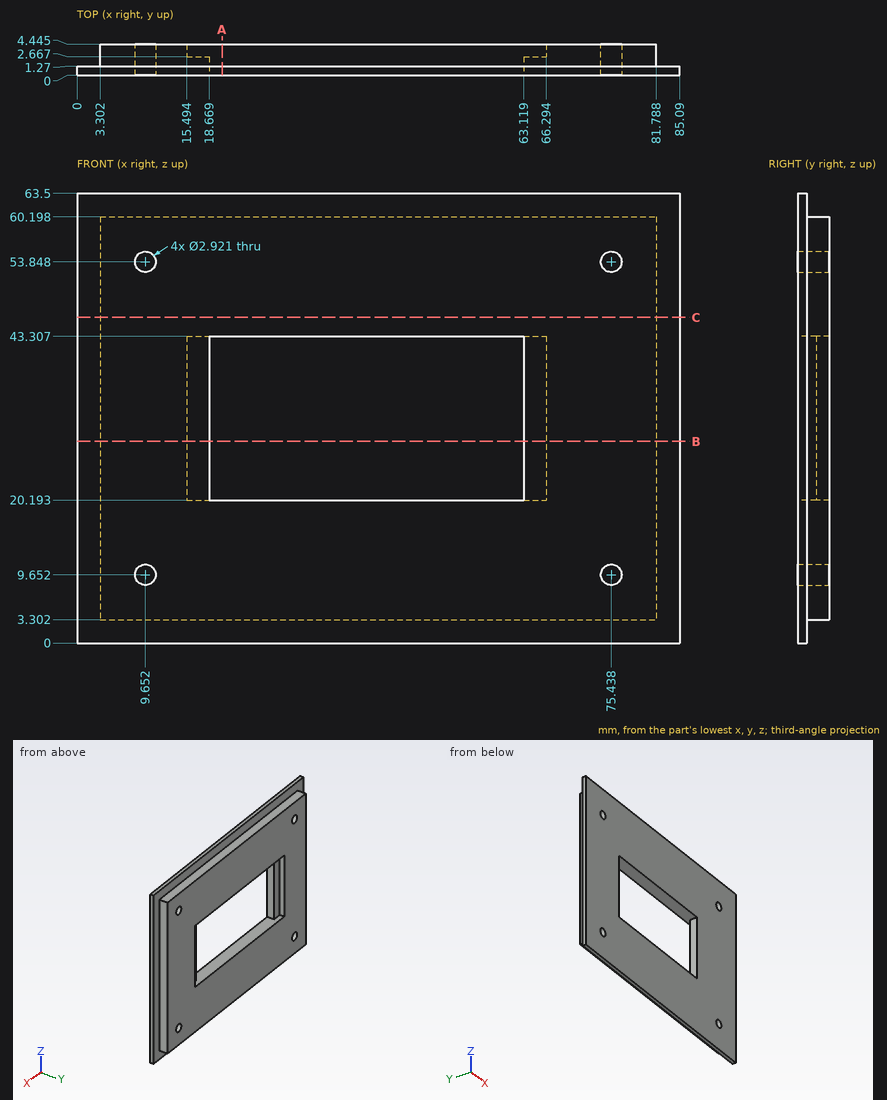
Here's the drawing with two shaded views (mm, measured from the low corner). I have some questions. Coordinates: 2 decimals unless noted, no trailing zeros. Write each loop counter-clockwise with the first axis right and the second up, starting at its lowest first coordinate (ties: lowest second). Pieces come first, ordered by that corner, then holes.
Item 1: I want a section at B-B on z = 28.5. Write out the boundary of the cut face in (x, y) (3 decimals).
Item 2: I want a section at C-C on z = 46. Write out the boundary of the cut face in (x, y) (3 decimals).
Item 3: I want a section at A-A on x = 20.5. Write out the boundary of the cut face in (y, z) (3 decimals).
Item 4: Will these pins go through, and if not, where does the flat tip stop? pin 1 (1.3 mm diameter, centred on x = 46.5, y = 2, fed in from +Z); pin 2 (1.6 mm diameter, centred on x = 65, z = 34.5, fed in from +Y); pin 3 (1 mm diameter, centred on x = 23.5, y = 2, fed in from -Z).
Item 5: If I drill on line 1 (X direction, y = 1, z = 21); line 2 (Z direction, x = 47.5, y = 1.75); line 3 (X direction, y = 3.6, z = 27), over which ranges is the centre line in solid material (lowest first)?
Findings below:
1. outline: (0, 0) - (18.669, 0) - (18.669, 2.667) - (15.494, 2.667) - (15.494, 4.445) - (3.302, 4.445) - (3.302, 1.27) - (0, 1.27) - close; (63.119, 0) - (85.09, 0) - (85.09, 1.27) - (81.788, 1.27) - (81.788, 4.445) - (66.294, 4.445) - (66.294, 2.667) - (63.119, 2.667) - close
2. outline: (0, 0) - (85.09, 0) - (85.09, 1.27) - (81.788, 1.27) - (81.788, 4.445) - (3.302, 4.445) - (3.302, 1.27) - (0, 1.27) - close
3. outline: (0, 0) - (1.27, 0) - (1.27, 3.302) - (4.445, 3.302) - (4.445, 20.193) - (0, 20.193) - close; (0, 43.307) - (4.445, 43.307) - (4.445, 60.198) - (1.27, 60.198) - (1.27, 63.5) - (0, 63.5) - close
4. pin 1: stops at z = 60.2
4. pin 2: stops at y = 2.67
4. pin 3: stops at z = 3.3
5. line 1: x = 0 to 18.67, 63.12 to 85.09
5. line 2: z = 3.3 to 20.19, 43.31 to 60.2
5. line 3: x = 3.3 to 15.49, 66.29 to 81.79
